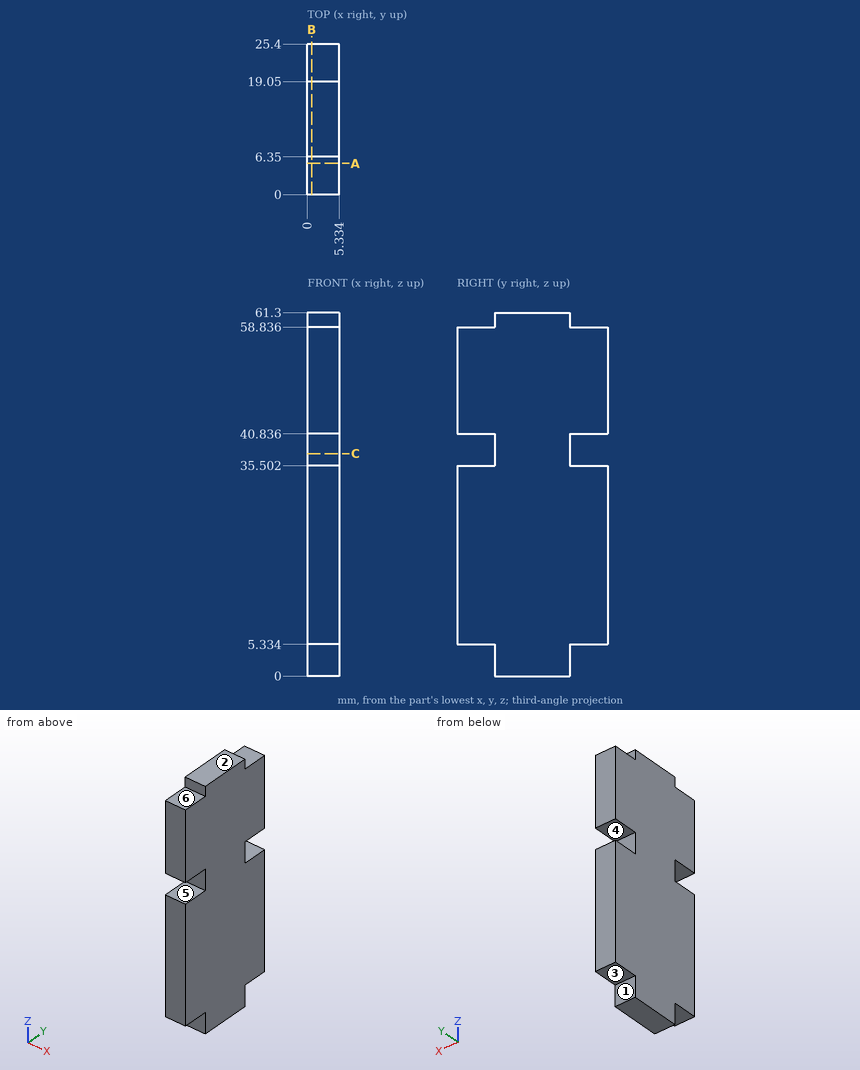
Geometry check sheet. Reference: drawing and pictorial views, mm from the part's lowest x, y, z. A direction names the side the tool comes from. Round coordinates to 2 decimals unless told otherwise and drop trailing zeros. Loops run counter-clockwise (first coordinate to the right, second up) from the corner with the lowest first, then second, coordinate; pieces in that order, holes last. Notation, with made-up numbers: M -6.75,54.25 L 6.25,54.25 A29 cw 6.25,86.25 Z; hole C -18.75,8 d2. An arc over 180 degrees is marked long. One line per item, written item: value.
(1) Sectioned sample at B-B, the plane x = 0.7. Record the cut outline in (y, z).
Computed values:
outline: M 0,5.33 L 6.35,5.33 L 6.35,0 L 19.05,0 L 19.05,5.33 L 25.4,5.33 L 25.4,35.5 L 19.05,35.5 L 19.05,40.84 L 25.4,40.84 L 25.4,58.84 L 19.05,58.84 L 19.05,61.3 L 6.35,61.3 L 6.35,58.84 L 0,58.84 L 0,40.84 L 6.35,40.84 L 6.35,35.5 L 0,35.5 Z
(2) Depth check by flat-ended pin: pin 1 Ø0.7 at (x, z) = (3.5, 60.5) entering from +Y; pin 2 Ø1 at (x, y) = (3.5, 20.5) entering from -Z; pin 3 Ø1.6 at (x, y) = (3, 20.5) entering from +Z; pin 4 Ø1.5 at (y, z) = (21.5, 40) entering from +X. Enter the tip coordinate at first touch or a pass-through.
Computed values:
pin 1: stops at y = 19.05
pin 2: stops at z = 5.33
pin 3: stops at z = 58.84
pin 4: passes through
(3) Sectioned sample at C-C, the plane z = 37.5. Record the cut outline in (x, y).
Computed values:
outline: M 0,6.35 L 5.33,6.35 L 5.33,19.05 L 0,19.05 Z
(4) Release check for a two-part mould opening along Z. For the marked faces 3, 4, 5 and 6 record: +Z half, -Z half, draft (parallel to the pull), parting line (faces both ways), or undercut.
Computed values:
face 3: -Z half
face 4: undercut
face 5: undercut
face 6: +Z half
(5) Access from +Z, -Z, +X, -X, +Y, -Y to the whole of each face (thin tool, end or side, straight path). Record for the marked faces 1 and 2.
Computed values:
face 1: -Z, +X, -X, +Y
face 2: +Z, +X, -X, +Y, -Y
(6) Thickness scan on line 1 (Z direction, x = 2.3, y = 19.5); line 2 (Y direction, x = 4.5, z = 40). Record the ranges inside material, lowest first.
Computed values:
line 1: z = 5.33 to 35.5, 40.84 to 58.84
line 2: y = 6.35 to 19.05
(7) Sectioned sample at A-A, the plane y = 5.25. Record the cut outline in (x, z).
Computed values:
outline: M 0,5.33 L 5.33,5.33 L 5.33,35.5 L 0,35.5 Z; M 0,40.84 L 5.33,40.84 L 5.33,58.84 L 0,58.84 Z
